```python
from build123d import *

# Parameters (mm, degrees)
SKETCH_1_W               = 8
SKETCH_1_H               = 8
EXTRUDE_1_DEPTH          = 20
EXTRUDE_2_DEPTH          = 2.5
CUT_EXTRUDE_1_DEPTH      = 41.91749234
CUT_EXTRUDE_1_DEPTH_BACK = 41.91749234
SKETCH_4_R               = 1.5
CUT_EXTRUDE_2_DEPTH      = 41.91749234
SKETCH_9_R               = 1.3
CUT_EXTRUDE_3_DEPTH      = 10
EXTRUDE_3_DEPTH          = 8
CUT_EXTRUDE_START        = -4
CUT_EXTRUDE_4_DEPTH      = 3.55


with BuildPart() as part:
    # 草图1 → 凸台-拉伸1 (new body)
    with BuildSketch(Plane(origin=(0, 0, 0), x_dir=(1, 0, 0), z_dir=(0, 1, 0))):
        Rectangle(SKETCH_1_W, SKETCH_1_H)
    extrude(amount=EXTRUDE_1_DEPTH)

    # 草图2 → 凸台-拉伸2 (add, symmetric)
    with BuildSketch(Plane(origin=(0, 0, 0), x_dir=(0, 0, -1), z_dir=(1, 0, 0))):
        Polygon((-4, 20), (26, 30.919107028), (26, 25.919107028), (-4, 15), align=None)
    extrude(amount=EXTRUDE_2_DEPTH, both=True)

    # 草图4 → 切除-拉伸1 (cut, two sides: drawn at the far end of the back side and taken through both)
    with BuildSketch(Plane(origin=(2.5, 0, 0), x_dir=(0, 0, -1), z_dir=(1, 0, 0)).offset(-CUT_EXTRUDE_1_DEPTH_BACK)):
        with Locations((-1.5, 18.409925586)):
            Circle(SKETCH_4_R)
        with Locations((23.5, 27.509181442)):
            Circle(SKETCH_4_R)
        with Locations((11, 22.959553514)):
            Circle(SKETCH_4_R)
    extrude(amount=CUT_EXTRUDE_1_DEPTH + CUT_EXTRUDE_1_DEPTH_BACK, mode=Mode.SUBTRACT)

    # 草图7 → 切除-拉伸2 (cut, through all)
    with BuildSketch(Plane.ZY.offset(2.5)):
        with BuildLine():
            Line((-26, 30.919107028), (-26, 25.919107028))
            Line((-26, 25.919107028), (-24.303484649, 25.301625938))
            ThreePointArc((-24.303484649, 25.301625938), (-25.707555519, 28.312666051), (-22.696515431, 29.716736975))
            Line((-22.696515431, 29.716736975), (-26, 30.919107028))
        make_face()
    extrude(amount=-CUT_EXTRUDE_2_DEPTH, mode=Mode.SUBTRACT)

    # 草图9 → 切除-拉伸3 (cut)
    with BuildSketch(Plane.XZ):
        with Locations(Location((0, 0, 0), (0, 0, 270))):
            Circle(SKETCH_9_R)
    extrude(amount=-CUT_EXTRUDE_3_DEPTH, mode=Mode.SUBTRACT)

    # 草图11 → 凸台-拉伸3 (add)
    with BuildSketch(Plane(origin=(4, 0, 0), x_dir=(0, 0, -1), z_dir=(1, 0, 0))):
        Polygon((-4, 20), (4, 20), (4, 22.911761874), align=None)
    extrude(amount=-EXTRUDE_3_DEPTH)

    # 草图12 → 切除-拉伸4 (cut)
    with BuildSketch(Plane.XZ.offset(CUT_EXTRUDE_START)):
        Polygon((2.840563324, 0), (1.420281662, 2.46), (-1.420281662, 2.46), (-2.840563324, 0), (-1.420281662, -2.46), (1.420281662, -2.46), align=None)
    extrude(amount=-CUT_EXTRUDE_4_DEPTH, mode=Mode.SUBTRACT)


solid = part.part
```
Work out the finished part from the listing and answer in its coordinate system (mm). A direction names the side the tool comes from. Round coordinates to 2 decimals unless told otherwise and drop trailing zeros. Write each loop counter-clockwise with the first axis right and the second up, starting at its lowest first coordinate (ties: lowest second). Pieces come first, ordered by that corner, then holes. Notation, with made-up numbers: (88.25, 58) -> (107.25, 58) arc R19 ccw to (107.25, 76) -> close; hole circle Ø6 at (87.25, -34). An arc over 180 degrees is marked (long way). Write each question's results on one line, items separated by ' | '.
Q1. Section C-C, the plane z = -11 is taken. Write down the section's boundary in (x, y), then the cut area to 3 significant figures.
Data:
outline: (-2.5, 20.46) -> (2.5, 20.46) -> (2.5, 21.46) -> (-2.5, 21.46) -> close; (-2.5, 24.46) -> (2.5, 24.46) -> (2.5, 25.46) -> (-2.5, 25.46) -> close | area: 10.0 mm^2
Q2. Section D-D, the plane x = 0 is taken. Write down the section's boundary in (y, z), then the cut area to 3 significant figures.
Data:
outline: (0, -4) -> (17.91, -4) -> (25.3, -24.3) arc R2.35 ccw to (29.72, -22.7) -> (20, 4) -> (0, 4) -> (0, 1.3) -> (4, 1.3) -> (4, 2.46) -> (7.55, 2.46) -> (7.55, 1.3) -> (10, 1.3) -> (10, -1.3) -> (7.55, -1.3) -> (7.55, -2.46) -> (4, -2.46) -> (4, -1.3) -> (0, -1.3) -> close; hole circle Ø3 at (18.41, 1.5); hole circle Ø3 at (22.96, -11); hole circle Ø3 at (27.51, -23.5) | area: 222 mm^2
Q3. Determine the mould class of faces 6 (the flat face through (-2, 0, 0)), 7 (the flat face through (0, 10, 4)), 8 (the flat face through (0, 11, -4)), 9 (the flat face through (2.14, 5.75, 1.21)) for opening direction Z: released by +Z, released by -Z, zero draft, split by the parting line, or undercut.
Data:
face 6: zero draft | face 7: released by +Z | face 8: released by -Z | face 9: undercut
Q4. Section A-A, the plane y = 5.75 is taken. Write down the section's boundary in (x, z).
Data:
outline: (-4, -4) -> (4, -4) -> (4, 4) -> (-4, 4) -> close; hole (-2.84, 0) -> (-1.42, -2.46) -> (1.42, -2.46) -> (2.84, 0) -> (1.42, 2.46) -> (-1.42, 2.46) -> close
Q5. Straight lines are drawn through the part: line 1 along X through (y, z) = (8.15, 0); line 2 along Y through (x, z) = (0, 1.5); line 3 along Z through (x, y) = (-0.25, 7). For each, find the intervals that lie inside material, in ascending order. Write a range as [from, to].
Data:
line 1: [-4, -1.3], [1.3, 4] | line 2: [0, 4], [7.55, 16.91], [19.91, 20.91] | line 3: [-4, -2.46], [2.46, 4]
Q6. Flat-ended cylindrical pins translate along their axes: P1, Ø13, axis at y = 24, z = -11, coming from the +X side; P2, Ø6, axis at y = 11.5, z = -9.5, coming from the +X side; P3, Ø3.5, axis at x = 0, z = 0, coming from the -Y side; P4, Ø2, axis at x = 1, y = 16.5, coming from the -Z side. Find the tip coordinate at first contact, or state that the pin passes through.
Data:
P1: x = 2.5 | P2: through | P3: y = 0 | P4: z = -4
Q7. Section B-B, the plane x = -2 is taken. Write down the section's boundary in (y, z), then the cut area to 3 significant figures.
Data:
outline: (0, -4) -> (17.91, -4) -> (25.3, -24.3) arc R2.35 ccw to (29.72, -22.7) -> (20, 4) -> (0, 4) -> close; hole (4, -1.46) -> (7.55, -1.46) -> (7.55, 1.46) -> (4, 1.46) -> close; hole circle Ø3 at (18.41, 1.5); hole circle Ø3 at (22.96, -11); hole circle Ø3 at (27.51, -23.5) | area: 246 mm^2
Q8. Which of the six approach directions +Z, -Z, +X, -X, +Y, -Y give full straight-line access (tool end or side, diameter ignored) to faces 1 (the cylindrical face through (0.39, 1.97, -1.24)), 2 (the flat face through (-2.5, 24, -14)), 3 (the cylindrical face through (-0.035, 28.996, -23.305)), 4 (the flat face through (2.5, 24, -14)), 5 (the flat face through (2.12, 5.75, -1.25))?
Data:
face 1: -Y | face 2: -Z, -X, +Y, -Y | face 3: +X, -X | face 4: -Z, +X, +Y, -Y | face 5: none
